Part model, mm, in its own coordinate system. A direction names the side the tool comes from. Give positions to 0.01 mm unless a question says otherwise; leave off trailing zeros. Write each loop counter-clockwise with the first axis right and the second up, starting at its lowest first coordinate (ties: lowest second). Pieces come first, ordered by that corner, then holes.
```python
from build123d import *
from OCP.BRepFilletAPI import BRepFilletAPI_MakeChamfer

# Parameters (mm, degrees)
BOSS_EXTRUDE1_DEPTH     = 6
CHAMFER1_SIZE           = 2.5
CHAMFER1_SIZE2          = 1.443375673
CUT_EXTRUDE1_DEPTH      = 43.848570571
CUT_EXTRUDE1_DEPTH_BACK = 28
SKETCH2_W               = 14
SKETCH2_H               = 6.892407629
SKETCH3_W               = 14
SKETCH3_H               = 20
CUT_EXTRUDE2_DEPTH      = 3.3
CHAMFER2_SIZE           = 4
HOLE1_D                 = 3
HOLE1_CBORE_D           = 4.1
HOLE1_CBORE_DEPTH       = 4
HOLE2_D                 = 3
HOLE2_CBORE_D           = 3.5
HOLE2_CBORE_DEPTH       = 20
FILLET2_R               = 5
CHAMFER3_SIZE           = 2
CHAMFER3_SIZE2          = 0.535898385


with BuildPart() as part:
    # Sketch1 → Boss-Extrude1 (new body)
    with BuildSketch(Plane.XY):
        with BuildLine():
            Line((-20, 30), (20, 30))
            ThreePointArc((20, 30), (27.071067812, 27.071067812), (30, 20))
            Line((30, 20), (30, -20))
            ThreePointArc((30, -20), (27.071067812, -27.071067812), (20, -30))
            Line((20, -30), (-20, -30))
            ThreePointArc((-20, -30), (-27.071067812, -27.071067812), (-30, -20))
            Line((-30, -20), (-30, 20))
            ThreePointArc((-30, 20), (-27.071067812, 27.071067812), (-20, 30))
        make_face()
    extrude(amount=BOSS_EXTRUDE1_DEPTH)

    # Chamfer1: one chamfer whose edges measure the first distance from different faces: ONE call of the kernel's chamfer builder (chamfer() names one face for all edges)
    chamfer1_edges_1 = [part.edges().sort_by_distance(p)[0] for p in [
        (0, 30, 0),
    ]]
    chamfer1_side_1 = [part.faces().sort_by_distance(p)[0] for p in [
        (0, 30, 3),
    ]]
    chamfer1_edges_2 = [part.edges().sort_by_distance(p)[0] for p in [
        (27.071067812, 27.071067812, 0),
    ]]
    chamfer1_side_2 = [part.faces().sort_by_distance(p)[0] for p in [
        (27.071067812, 27.071067812, 3),
    ]]
    chamfer1_edges_3 = [part.edges().sort_by_distance(p)[0] for p in [
        (30, 0, 0),
    ]]
    chamfer1_side_3 = [part.faces().sort_by_distance(p)[0] for p in [
        (30, 0, 3),
    ]]
    chamfer1_edges_4 = [part.edges().sort_by_distance(p)[0] for p in [
        (27.071067812, -27.071067812, 0),
    ]]
    chamfer1_side_4 = [part.faces().sort_by_distance(p)[0] for p in [
        (27.071067812, -27.071067812, 3),
    ]]
    chamfer1_edges_5 = [part.edges().sort_by_distance(p)[0] for p in [
        (0, -30, 0),
    ]]
    chamfer1_side_5 = [part.faces().sort_by_distance(p)[0] for p in [
        (0, -30, 3),
    ]]
    chamfer1_edges_6 = [part.edges().sort_by_distance(p)[0] for p in [
        (-27.071067812, -27.071067812, 0),
    ]]
    chamfer1_side_6 = [part.faces().sort_by_distance(p)[0] for p in [
        (-27.071067812, -27.071067812, 3),
    ]]
    chamfer1_edges_7 = [part.edges().sort_by_distance(p)[0] for p in [
        (-30, 0, 0),
    ]]
    chamfer1_side_7 = [part.faces().sort_by_distance(p)[0] for p in [
        (-30, 0, 3),
    ]]
    chamfer1_edges_8 = [part.edges().sort_by_distance(p)[0] for p in [
        (-27.071067812, 27.071067812, 0),
    ]]
    chamfer1_side_8 = [part.faces().sort_by_distance(p)[0] for p in [
        (-27.071067812, 27.071067812, 3),
    ]]
    chamfer1 = BRepFilletAPI_MakeChamfer(part.part.solid().wrapped)
    for e in chamfer1_edges_1:
        chamfer1.Add(CHAMFER1_SIZE, CHAMFER1_SIZE2, e.wrapped, chamfer1_side_1[0].wrapped)  # the first distance lies on this face
    for e in chamfer1_edges_2:
        chamfer1.Add(CHAMFER1_SIZE, CHAMFER1_SIZE2, e.wrapped, chamfer1_side_2[0].wrapped)  # the first distance lies on this face
    for e in chamfer1_edges_3:
        chamfer1.Add(CHAMFER1_SIZE, CHAMFER1_SIZE2, e.wrapped, chamfer1_side_3[0].wrapped)  # the first distance lies on this face
    for e in chamfer1_edges_4:
        chamfer1.Add(CHAMFER1_SIZE, CHAMFER1_SIZE2, e.wrapped, chamfer1_side_4[0].wrapped)  # the first distance lies on this face
    for e in chamfer1_edges_5:
        chamfer1.Add(CHAMFER1_SIZE, CHAMFER1_SIZE2, e.wrapped, chamfer1_side_5[0].wrapped)  # the first distance lies on this face
    for e in chamfer1_edges_6:
        chamfer1.Add(CHAMFER1_SIZE, CHAMFER1_SIZE2, e.wrapped, chamfer1_side_6[0].wrapped)  # the first distance lies on this face
    for e in chamfer1_edges_7:
        chamfer1.Add(CHAMFER1_SIZE, CHAMFER1_SIZE2, e.wrapped, chamfer1_side_7[0].wrapped)  # the first distance lies on this face
    for e in chamfer1_edges_8:
        chamfer1.Add(CHAMFER1_SIZE, CHAMFER1_SIZE2, e.wrapped, chamfer1_side_8[0].wrapped)  # the first distance lies on this face
    add(Compound.cast(chamfer1.Shape()), mode=Mode.REPLACE)

    # Sketch2 → Cut-Extrude1 (cut, two sides: drawn at the far end of the back side and taken through both)
    with BuildSketch(Plane(origin=(0, 0, 0), x_dir=(1, 0, 0), z_dir=(0, 1, 0)).offset(-CUT_EXTRUDE1_DEPTH_BACK)):
        with Locations((0, -7.446203815)):
            Rectangle(SKETCH2_W, SKETCH2_H)
    extrude(amount=CUT_EXTRUDE1_DEPTH + CUT_EXTRUDE1_DEPTH_BACK, mode=Mode.SUBTRACT)

    # Sketch3 → Cut-Extrude2 (cut)
    with BuildSketch(Plane.XY.offset(4)):
        Rectangle(SKETCH3_W, SKETCH3_H)
    extrude(amount=-CUT_EXTRUDE2_DEPTH, mode=Mode.SUBTRACT)

    # Chamfer2
    # the kernel refuses this chamfer: 4 mm, written as the material it takes off along each edge
    with BuildSketch(Plane(origin=(-7, 10, 4), x_dir=(0, 0.9996219169112968, 0.02749587661058627), z_dir=(1, 0, 0))) as chamfer2_piece_1_section:
        Polygon((CHAMFER2_SIZE * 0.999621916911, -CHAMFER2_SIZE * 0.0274958766106), (-CHAMFER2_SIZE * 0.0274958766106, -CHAMFER2_SIZE * 0.999621916911), (0, 0), align=None)
    chamfer2_piece_1 = extrude(amount=14, mode=Mode.PRIVATE)
    chamfer2_piece_1 = split(chamfer2_piece_1, bisect_by=Plane(origin=(0, 11.371649583, 0.7), z_dir=(0, 0, 1)), keep=Keep.TOP, mode=Mode.PRIVATE)
    add(chamfer2_piece_1, mode=Mode.SUBTRACT)
    with BuildSketch(Plane(origin=(7, -10, 4), x_dir=(0, -0.9996219169112968, 0.02749587661058627), z_dir=(-1, 0, 0))) as chamfer2_piece_2_section:
        Polygon((CHAMFER2_SIZE * 0.999621916911, -CHAMFER2_SIZE * 0.0274958766106), (-CHAMFER2_SIZE * 0.0274958766106, -CHAMFER2_SIZE * 0.999621916911), (0, 0), align=None)
    chamfer2_piece_2 = extrude(amount=14, mode=Mode.PRIVATE)
    chamfer2_piece_2 = split(chamfer2_piece_2, bisect_by=Plane(origin=(0, -11.371649583, 0.7), z_dir=(0, 0, 1)), keep=Keep.TOP, mode=Mode.PRIVATE)
    add(chamfer2_piece_2, mode=Mode.SUBTRACT)

    # Hole1 (through all)
    with Locations(Plane(origin=(0, 0, 0), x_dir=(-1, 0, 0), z_dir=(0, 0, -1))):
        with Locations((20, -20), (-20, -20), (-20, 20), (20, 20)):
            CounterBoreHole(HOLE1_D / 2, HOLE1_CBORE_D / 2, HOLE1_CBORE_DEPTH)

    # Hole2 (through all)
    with Locations(Plane.XY.offset(4)):
        with Locations((3, 20), (-3, 20), (0, -20)):
            CounterBoreHole(HOLE2_D / 2, HOLE2_CBORE_D / 2, HOLE2_CBORE_DEPTH)

    # Fillet2
    fillet2_edges = [part.edges().sort_by_distance(p)[0] for p in [
        (-7, -28, 5),
        (7, -28, 5),
    ]]
    fillet(fillet2_edges, radius=FILLET2_R)

    # Chamfer3: one chamfer whose edges measure the first distance from different faces: ONE call of the kernel's chamfer builder (chamfer() names one face for all edges)
    chamfer3_edges_1 = [part.edges().sort_by_distance(p)[0] for p in [
        (22.05, 20, 0),
    ]]
    chamfer3_side_1 = [part.faces().sort_by_distance(p)[0] for p in [
        (22.05, 20, 2),
    ]]
    chamfer3_edges_2 = [part.edges().sort_by_distance(p)[0] for p in [
        (22.05, -20, 0),
    ]]
    chamfer3_side_2 = [part.faces().sort_by_distance(p)[0] for p in [
        (22.05, -20, 2),
    ]]
    chamfer3_edges_3 = [part.edges().sort_by_distance(p)[0] for p in [
        (-17.95, -20, 0),
    ]]
    chamfer3_side_3 = [part.faces().sort_by_distance(p)[0] for p in [
        (-17.95, -20, 2),
    ]]
    chamfer3_edges_4 = [part.edges().sort_by_distance(p)[0] for p in [
        (-17.95, 20, 0),
    ]]
    chamfer3_side_4 = [part.faces().sort_by_distance(p)[0] for p in [
        (-17.95, 20, 2),
    ]]
    chamfer3 = BRepFilletAPI_MakeChamfer(part.part.solid().wrapped)
    for e in chamfer3_edges_1:
        chamfer3.Add(CHAMFER3_SIZE, CHAMFER3_SIZE2, e.wrapped, chamfer3_side_1[0].wrapped)  # the first distance lies on this face
    for e in chamfer3_edges_2:
        chamfer3.Add(CHAMFER3_SIZE, CHAMFER3_SIZE2, e.wrapped, chamfer3_side_2[0].wrapped)  # the first distance lies on this face
    for e in chamfer3_edges_3:
        chamfer3.Add(CHAMFER3_SIZE, CHAMFER3_SIZE2, e.wrapped, chamfer3_side_3[0].wrapped)  # the first distance lies on this face
    for e in chamfer3_edges_4:
        chamfer3.Add(CHAMFER3_SIZE, CHAMFER3_SIZE2, e.wrapped, chamfer3_side_4[0].wrapped)  # the first distance lies on this face
    add(Compound.cast(chamfer3.Shape()), mode=Mode.REPLACE)


solid = part.part
```
1) Two-plate mould, pull along X, no slides. Class faces 4 (the face through (26.99, 27.15, 4.23)), 5 (the face through (0.28, -29.268, 1.233)), 6 (the face through (18.89, -18.99, 5.01)): +X half, -X half, draft (parallel to the pull), parting line (faces both ways), or undercut.
Answers follow:
face 4: +X half
face 5: draft
face 6: undercut
2) 3-axis set-ups, long thin cutter, end or side, ignore diameter. For faces 1 (the face through (0, -28, 5)), 2 (the face through (0, -12, 2)), 3 (the face through (2.772, 21.735, 2.028)): which of +Z, -Z, +X, -X, +Y, -Y reach the whole face in a straight line?
Answers follow:
face 1: +Z, +Y
face 2: +Z
face 3: +Z, -Z
3) Pin check, flat tips, straight feed: pin 1 Ø1.5 at (y, z) = (22.5, 1.5) entering from -X; pin 2 Ø3 at (y, z) = (-21, 1) entering from -X; pin 3 Ø7 at (x, y) = (-2, 3.5) entering from +Z. Stop position of each tip, or through.
Answers follow:
pin 1: stops at x = -29.57
pin 2: stops at x = -29.96
pin 3: stops at z = 0.7
4) Wall check: L1, parallel to Y at x = 20, z = 5.1; L2, parallel to X at y = 8, z = 2.75; L3, parallel to Y at x = -18.5, z = 1.25. Give the ranges that are in metal, low to high.
Answers follow:
L1: y = -30 to -21.5, -18.5 to 18.5, 21.5 to 30
L2: x = -30 to -7, 7 to 30
L3: y = -29.28 to -21.68, -18.32 to 18.32, 21.68 to 29.28
5) Saw through at B-B, the plane z = 5. Write the cut outline in (x, y), then the cut area to 3 significant figures.
Answers follow:
outline: (-30, -20) arc R10 ccw to (-20, -30) - (20, -30) arc R10 ccw to (30, -20) - (30, 20) arc R10 ccw to (20, 30) - (7, 30) - (7, -23) arc R5 cw to (2, -28) - (-2, -28) arc R5 cw to (-7, -23) - (-7, 30) - (-20, 30) arc R10 ccw to (-30, 20) - close; hole circle Ø3 at (-20, -20); hole circle Ø3 at (-20, 20); hole circle Ø3 at (20, -20); hole circle Ø3 at (20, 20)
area: 2,680 mm2
6) Saw through at A-A, the plane y = -2. Write the cut outline in (x, z).
Answers follow:
outline: (-30, 2.5) - (-28.56, 0) - (28.56, 0) - (30, 2.5) - (30, 6) - (7, 6) - (7, 0.7) - (-7, 0.7) - (-7, 6) - (-30, 6) - close
7) Saw through at C-C, the plane x = 3. Write the cut outline in (y, z), then the cut area to 3 significant figures.
Answers follow:
outline: (-30, 2.5) - (-28.56, 0) - (18.25, 0) - (18.25, 4) - (14, 4) - (10.7, 0.7) - (-10.7, 0.7) - (-14, 4) - (-27.9, 4) - (-27.9, 6) - (-30, 6) - close; (21.75, 0) - (28.56, 0) - (30, 2.5) - (30, 4) - (21.75, 4) - close
area: 145 mm2
